Input: part model. Units: mm. Frame: model coordinates. A direction names the side the tool comes from. Give positions to 0.01 mm unless a question says otherwise; leave off trailing zeros. Write each loop counter-clockwise with the first axis right and the second up, starting at its lowest first coordinate (ties: lowest second). Pieces come first, ordered by that corner, then holes. Notation, with made-up numbers: (61, -27.5) -> (120, -27.5) arc R27 ccw to (120, -10.5) -> close; hole circle Ø9 at (-0.75, -16). An arc over 180 degrees is marked (long way). Return JSON: item names as keys, results as strings. Group by question number.
Item 1: Pin query (flat end, axial travel): P1, Ø5, axis at x = -22, z = 26.5, coming from the -Y side; P2, Ø1, axis at x = -11, y = 36.5, coming from the +Z side; P3, Ø5, axis at x = -26.45, y = 36.41, coming from the +Z side; P4, Ø12, axis at y = -4.5, z = 14.5, coming from the +X side. Return the tip coordinate at first contact, or that it passes through.
Item 2: Section B-B, the plane x = -6. Return loops of the section in (y, z).
Item 3: Section C-C, the plane y = 36.5. Return loops of the section in (x, z).
Item 4: Section A-A, the plane z = 85. Return loops of the section in (x, y), then the cut area to 3 significant figures.
Item 5: Section D-D, the plane x = 43. Return loops of the section in (y, z), then the cut area to 3 significant figures.
Item 6: Line query: line 1 (Y direction, x = 0, z = 5); line 2 (Y direction, x = 0, z = 11); line 3 (X direction, y = -20.5, z = 61). Output: solid intervals per line, ascending. Write a range as [from, to].
Item 7: Set-up query: faces 1 (the face through (24, -22, 67)), 2 (the face through (-23, -30, 68)), 3 (the face through (-22, -12, 68)), 4 (the face through (0, -11, 67)), 5 (the face through (23, -13, 68)). Return all of +Z, -Z, +X, -X, +Y, -Y with unobstructed straight access to the full face (end or side cutting, diameter ignored); none if empty.
Item 8: Mould query, pull axis X, two halves, no side actions, for faces 6 (the face through (41.1, -11.43, 4.93)), 7 (the face through (-8.67, 39.05, 24.79)), 8 (the face through (-4, -41, 10)). Classes: released by +X, released by -X, zero draft, split by the parting line, or undercut.
Solid Edge part; units mm, degrees
sketch "Sketch1" plane through (0, 0, 0) normal (0, 0, 1) x (1, 0, 0)
  circle A0 centre (0, 0) radius 50
  circle A1 centre (0, 0) radius 10
extrude "Protrusion1" add sketch "Sketch1" along normal blind 10
hole "Bohrung_9" at (0, 45, 0) direction (0, 0, 1) diameter 6 end up to next
pattern_circular "Pattern1" count 10 over 360 about axis through (0, 0, 10) along (0, 0, -1) of "Bohrung_9"
sketch "Sketch2" plane through (0, 0, 10) normal (0, 0, 1) x (1, 0, 0)
  circle A0 centre (0, 0) radius 40
  circle A1 centre (0, 0) radius 10
extrude "Extrusionsausprägung_9" add sketch "Sketch2" along normal blind 30
sketch "Sketch3" plane through (0, 0, 40) normal (0, 0, 1) x (-1, 0, 0)
  line L0 (24, 11) -> (24, 32)
  line L1 (24, 32) -> (-24, 32)
  line L2 (-24, 32) -> (-24, 11)
  line L3 (-24, 11) -> (24, 11)
extrude "Extrusionsausprägung_10" add sketch "Sketch3" along normal blind 60
sketch "Sketch4" plane through (24, -63.1755, 70) normal (1, 0, 0) x (0, 1, 0)
  circle A0 centre (41.6755, 15) radius 3
extrude "Cutout1" cut sketch "Sketch4" against normal up to next
fillet "Verrundung_5" radius 5 8 edges at (24, -32, 70) (24, -11, 70) (24, -21.5, 100) (0, -32, 100) (0, -11, 100) (-24, -32, 70) (-24, -21.5, 100) (-24, -11, 70)
Answer below:
{
 "1": {"P1": "stops at y = -34.92", "P2": "stops at z = 40", "P3": "passes through", "P4": "stops at x = 50"},
 "2": {"outline": "(-49.64, 0) -> (-8, 0) -> (-8, 40) -> (-11, 40) -> (-11, 95) arc R5 ccw to (-16, 100) -> (-27, 100) arc R5 ccw to (-32, 95) -> (-32, 40) -> (-39.55, 40) -> (-39.55, 10) -> (-49.64, 10) -> close; (8, 0) -> (49.64, 0) -> (49.64, 10) -> (39.55, 10) -> (39.55, 40) -> (8, 40) -> close; hole circle Ø6 at (-21.5, 85)"},
 "3": {"outline": "(-34.17, 0) -> (-29.45, 0) -> (-29.45, 10) -> (-34.17, 10) -> close; (-23.45, 0) -> (23.45, 0) -> (23.45, 10) -> (16.36, 10) -> (16.36, 40) -> (-16.36, 40) -> (-16.36, 10) -> (-23.45, 10) -> close; (29.45, 0) -> (34.17, 0) -> (34.17, 10) -> (29.45, 10) -> close"},
 "4": {"outline": "(-24, -27) arc R5 ccw to (-19, -32) -> (19, -32) arc R5 ccw to (24, -27) -> (24, -24.5) -> (-24, -24.5) -> close; (-24, -18.5) -> (24, -18.5) -> (24, -16) arc R5 ccw to (19, -11) -> (-19, -11) arc R5 ccw to (-24, -16) -> close", "area": "699 mm2"},
 "5": {"outline": "(-25.51, 0) -> (-16.9, 0) -> (-16.9, 10) -> (-25.51, 10) -> close; (-10.91, 0) -> (10.91, 0) -> (10.91, 10) -> (-10.91, 10) -> close; (16.9, 0) -> (25.51, 0) -> (25.51, 10) -> (16.9, 10) -> close", "area": "391 mm2"},
 "6": {"line 1": "y = [-50, -48], [-42, -10], [10, 42], [48, 50]", "line 2": "y = [-40, -10], [10, 40]", "line 3": "x = [-24, 24]"},
 "7": {"face 1": "+Z, +X, +Y, -Y", "face 2": "+Z, -X, -Y", "face 3": "+Z, -X, +Y", "face 4": "+Z, +X, -X, +Y", "face 5": "+Z, +X, +Y"},
 "8": {"face 6": "undercut", "face 7": "split by the parting line", "face 8": "zero draft"}
}
